from build123d import *
from build123d.topology import SkipClean

# Parameters (mm, degrees)
BOSS_EXTRUDE1_DEPTH = 5
SKETCH3_W           = 36.405926788
SKETCH3_H           = 27.783470444
CUT_EXTRUDE1_DEPTH  = 36
CUT_EXTRUDE2_REACH  = 86.1
SKETCH4_R           = 7.5
BOSS_EXTRUDE2_REACH = 86.1
SKETCH5_R           = 1
RIB2_REACH          = 70.337
SKETCH6_WALL_W      = 155.225095754
SKETCH6_WALL_H      = 3
RIB3_REACH          = 83.817
SKETCH7_WALL_W      = 192.357197592
SKETCH7_WALL_H      = 3
RIB4_REACH          = 83.817
SKETCH9_WALL_W      = 192.357197592
SKETCH9_WALL_H      = 3
SKETCH10_R          = 1.5
CUT_EXTRUDE3_DEPTH  = 5


with BuildPart() as part:
    # Sketch1 → Boss-Extrude1 (new body)
    with BuildSketch(Plane(origin=(0, 0, 0), x_dir=(1, 0, 0), z_dir=(0, 1, 0))):
        with BuildLine():
            Line((35, 20), (-35, 20))
            ThreePointArc((-35, 20), (-45.606601718, 15.606601718), (-50, 5))
            Line((-50, 5), (-50, -5))
            ThreePointArc((-50, -5), (-45.606601718, -15.606601718), (-35, -20))
            Line((-35, -20), (35, -20))
            ThreePointArc((35, -20), (45.606601718, -15.606601718), (50, -5))
            Line((50, -5), (50, 5))
            ThreePointArc((50, 5), (45.606601718, 15.606601718), (35, 20))
        make_face()
    extrude(amount=BOSS_EXTRUDE1_DEPTH)

    # Sketch2 → Revolve2 (revolve)
    with SkipClean():  # the faces are left unmerged after this step: merging them gives an invalid solid
        with BuildSketch(Plane.XY, mode=Mode.PRIVATE) as revolve2_sk:
            Polygon((-30, 0), (12.071067812, 42.071067812), (19.142135624, 35), (-15.857864376, 0), align=None)
        revolve(revolve2_sk.sketch.rotate(Axis((19.142135624, 35, 0), (-0.7071067811865515, -0.7071067811865436, 0)), 180), axis=Axis((19.142135624, 35, 0), (-0.7071067811865515, -0.7071067811865436, 0)))

    # Sketch3 → Cut-Extrude1 (cut)
    with BuildSketch(Plane.XZ):
        with Locations((-14.157860418, 0)):
            Rectangle(SKETCH3_W, SKETCH3_H)
    extrude(amount=CUT_EXTRUDE1_DEPTH, mode=Mode.SUBTRACT)

    # Cut-Extrude2: up to this plane
    cut_extrude2_end = Plane(origin=(-35, 5, -5), z_dir=(0, 1, 0))
    # Sketch4 → Cut-Extrude2 (cut, up to the surface)
    with BuildSketch(Plane(origin=(27.071067812, 27.071067812, 0), x_dir=(0, 0, -1), z_dir=(0.7071067811865513, 0.7071067811865438, 0)), mode=Mode.PRIVATE) as cut_extrude2_sk1:
        with Locations(Location((0, 11.213203436, 0), (0, 0, 90))):
            Circle(SKETCH4_R)
    cut_extrude2_tool1 = split(extrude(cut_extrude2_sk1.sketch, amount=-CUT_EXTRUDE2_REACH, mode=Mode.PRIVATE), bisect_by=cut_extrude2_end, keep=Keep.BOTH, mode=Mode.PRIVATE)
    add(cut_extrude2_tool1.solids().sort_by_distance((19.142136, 35, 0))[0], mode=Mode.SUBTRACT)

    # Boss-Extrude2: up to this plane
    boss_extrude2_end = Plane(origin=(-35, 5, -5), z_dir=(0, 1, 0))
    # Sketch5 → Boss-Extrude2 (add, up to the surface)
    with BuildSketch(Plane(origin=(27.071067812, 27.071067812, 0), x_dir=(0, 0, -1), z_dir=(0.7071067811865513, 0.7071067811865438, 0)), mode=Mode.PRIVATE) as boss_extrude2_sk1:
        with Locations((7.5, 11.213203436)):
            Circle(SKETCH5_R)
    boss_extrude2_tool1 = split(extrude(boss_extrude2_sk1.sketch, amount=-BOSS_EXTRUDE2_REACH, mode=Mode.PRIVATE), bisect_by=boss_extrude2_end, keep=Keep.BOTH, mode=Mode.PRIVATE)
    add(boss_extrude2_tool1.solids().sort_by_distance((19.142136, 35, -7.5))[0])
    # Sketch5 → Boss-Extrude2 (add, up to the surface)
    with BuildSketch(Plane(origin=(27.071067812, 27.071067812, 0), x_dir=(0, 0, -1), z_dir=(0.7071067811865513, 0.7071067811865438, 0)), mode=Mode.PRIVATE) as boss_extrude2_sk2:
        with Locations((5.303300859, 5.909902577)):
            Circle(SKETCH5_R)
    boss_extrude2_tool2 = split(extrude(boss_extrude2_sk2.sketch, amount=-BOSS_EXTRUDE2_REACH, mode=Mode.PRIVATE), bisect_by=boss_extrude2_end, keep=Keep.BOTH, mode=Mode.PRIVATE)
    add(boss_extrude2_tool2.solids().sort_by_distance((22.892136, 31.25, -5.303301))[0])
    # Sketch5 → Boss-Extrude2 (add, up to the surface)
    with BuildSketch(Plane(origin=(27.071067812, 27.071067812, 0), x_dir=(0, 0, -1), z_dir=(0.7071067811865513, 0.7071067811865438, 0)), mode=Mode.PRIVATE) as boss_extrude2_sk3:
        with Locations((0, 3.713203436)):
            Circle(SKETCH5_R)
    boss_extrude2_tool3 = split(extrude(boss_extrude2_sk3.sketch, amount=-BOSS_EXTRUDE2_REACH, mode=Mode.PRIVATE), bisect_by=boss_extrude2_end, keep=Keep.BOTH, mode=Mode.PRIVATE)
    add(boss_extrude2_tool3.solids().sort_by_distance((24.445436, 29.696699, 0))[0])
    # Sketch5 → Boss-Extrude2 (add, up to the surface)
    with BuildSketch(Plane(origin=(27.071067812, 27.071067812, 0), x_dir=(0, 0, -1), z_dir=(0.7071067811865513, 0.7071067811865438, 0)), mode=Mode.PRIVATE) as boss_extrude2_sk4:
        with Locations((-5.303300859, 5.909902577)):
            Circle(SKETCH5_R)
    boss_extrude2_tool4 = split(extrude(boss_extrude2_sk4.sketch, amount=-BOSS_EXTRUDE2_REACH, mode=Mode.PRIVATE), bisect_by=boss_extrude2_end, keep=Keep.BOTH, mode=Mode.PRIVATE)
    add(boss_extrude2_tool4.solids().sort_by_distance((22.892136, 31.25, 5.303301))[0])
    # Sketch5 → Boss-Extrude2 (add, up to the surface)
    with BuildSketch(Plane(origin=(27.071067812, 27.071067812, 0), x_dir=(0, 0, -1), z_dir=(0.7071067811865513, 0.7071067811865438, 0)), mode=Mode.PRIVATE) as boss_extrude2_sk5:
        with Locations((-7.5, 11.213203436)):
            Circle(SKETCH5_R)
    boss_extrude2_tool5 = split(extrude(boss_extrude2_sk5.sketch, amount=-BOSS_EXTRUDE2_REACH, mode=Mode.PRIVATE), bisect_by=boss_extrude2_end, keep=Keep.BOTH, mode=Mode.PRIVATE)
    add(boss_extrude2_tool5.solids().sort_by_distance((19.142136, 35, 7.5))[0])
    # Sketch5 → Boss-Extrude2 (add, up to the surface)
    with BuildSketch(Plane(origin=(27.071067812, 27.071067812, 0), x_dir=(0, 0, -1), z_dir=(0.7071067811865513, 0.7071067811865438, 0)), mode=Mode.PRIVATE) as boss_extrude2_sk6:
        with Locations((-5.303300859, 16.516504294)):
            Circle(SKETCH5_R)
    boss_extrude2_tool6 = split(extrude(boss_extrude2_sk6.sketch, amount=-BOSS_EXTRUDE2_REACH, mode=Mode.PRIVATE), bisect_by=boss_extrude2_end, keep=Keep.BOTH, mode=Mode.PRIVATE)
    add(boss_extrude2_tool6.solids().sort_by_distance((15.392136, 38.75, 5.303301))[0])
    # Sketch5 → Boss-Extrude2 (add, up to the surface)
    with BuildSketch(Plane(origin=(27.071067812, 27.071067812, 0), x_dir=(0, 0, -1), z_dir=(0.7071067811865513, 0.7071067811865438, 0)), mode=Mode.PRIVATE) as boss_extrude2_sk7:
        with Locations((0, 18.713203436)):
            Circle(SKETCH5_R)
    boss_extrude2_tool7 = split(extrude(boss_extrude2_sk7.sketch, amount=-BOSS_EXTRUDE2_REACH, mode=Mode.PRIVATE), bisect_by=boss_extrude2_end, keep=Keep.BOTH, mode=Mode.PRIVATE)
    add(boss_extrude2_tool7.solids().sort_by_distance((13.838835, 40.303301, 0))[0])
    # Sketch5 → Boss-Extrude2 (add, up to the surface)
    with BuildSketch(Plane(origin=(27.071067812, 27.071067812, 0), x_dir=(0, 0, -1), z_dir=(0.7071067811865513, 0.7071067811865438, 0)), mode=Mode.PRIVATE) as boss_extrude2_sk8:
        with Locations((5.303300859, 16.516504294)):
            Circle(SKETCH5_R)
    boss_extrude2_tool8 = split(extrude(boss_extrude2_sk8.sketch, amount=-BOSS_EXTRUDE2_REACH, mode=Mode.PRIVATE), bisect_by=boss_extrude2_end, keep=Keep.BOTH, mode=Mode.PRIVATE)
    add(boss_extrude2_tool8.solids().sort_by_distance((15.392136, 38.75, -5.303301))[0])

    # Sketch6 wall → Rib2 (add, up to next)
    with BuildSketch(Plane(origin=(26.502692564, 15.5, 0), x_dir=(0.422618261725, -0.906307787044, 0), z_dir=(0.906307787044, 0.422618261725, 0)), mode=Mode.PRIVATE) as rib2_sk1:
        Rectangle(SKETCH6_WALL_W, SKETCH6_WALL_H)
    rib2_tool1 = extrude(rib2_sk1.sketch, amount=-RIB2_REACH, mode=Mode.PRIVATE) - part.part
    add(rib2_tool1.solids().sort_by_distance((26.502692564, 15.5, 0))[0])

    # Sketch7 wall → Rib3 (add, up to next)
    with BuildSketch(Plane(origin=(17.261595026, 14.641447257, 10.75), x_dir=(0, -0.721603754863, 0.69230630574), z_dir=(0, -0.69230630574, -0.721603754863)), mode=Mode.PRIVATE) as rib3_sk1:
        Rectangle(SKETCH7_WALL_W, SKETCH7_WALL_H)
    rib3_tool1 = extrude(rib3_sk1.sketch, amount=RIB3_REACH, mode=Mode.PRIVATE) - part.part
    add(rib3_tool1.solids().sort_by_distance((17.261595026, 14.641447257, 10.75))[0])

    # Sketch9 wall → Rib4 (add, up to next)
    with BuildSketch(Plane(origin=(17.261595026, 14.641447257, -10.75), x_dir=(0, -0.721603754863, -0.69230630574), z_dir=(0, 0.69230630574, -0.721603754863)), mode=Mode.PRIVATE) as rib4_sk1:
        Rectangle(SKETCH9_WALL_W, SKETCH9_WALL_H)
    rib4_tool1 = extrude(rib4_sk1.sketch, amount=-RIB4_REACH, mode=Mode.PRIVATE) - part.part
    add(rib4_tool1.solids().sort_by_distance((17.261595026, 14.641447257, -10.75))[0])

    # Sketch10 → Cut-Extrude3 (cut)
    with BuildSketch(Plane.XZ):
        with Locations(Location((-40, 0, 0), (0, 0, 270))):
            Circle(SKETCH10_R)
        with Locations(Location((40, 15, 0), (0, 0, 270))):
            Circle(SKETCH10_R)
        with Locations(Location((40, -15, 0), (0, 0, 270))):
            Circle(SKETCH10_R)
    extrude(amount=-CUT_EXTRUDE3_DEPTH, mode=Mode.SUBTRACT)


solid = part.part
The listing builds one solid part. Answer for the finished solid, in the listing's coordinates (mm). A direction names the side the tool comes from. Give positions to 0.01 mm unless a question says otherwise; leave off trailing zeros. Order: outer loops, then holes, each group sorted by start corner. A loop starts at its lowest first (then second) coordinate and runs counter-clockwise, first axis right, second up. Notation, with made-up numbers: (-11, 52.25) - (33, 52.25) arc R20 cw to (33, 61.25) - close; hole circle Ø5 at (69, 4.25). An arc over 180 degrees is marked (long way). Use one line per item in the form item = value.
1) Find section D-D on z = 15. Determine the outline of the cut face in (x, y).
Verdict:
outline = (-46.18, 0) - (38.5, 0) - (38.5, 5) - (18.76, 5) - (18.76, 10.21) - (15.76, 10.21) - (15.76, 5) - (-46.18, 5) - close; (41.5, 0) - (46.18, 0) - (46.18, 5) - (41.5, 5) - close
2) Find section B-B on x = 40. Determine the outline of the cut face in (y, z), and give its area (3 significant figures).
Verdict:
outline = (0, -19.14) - (5, -19.14) - (5, -16.5) - (0, -16.5) - close; (0, -13.5) - (5, -13.5) - (5, 13.5) - (0, 13.5) - close; (0, 16.5) - (5, 16.5) - (5, 19.14) - (0, 19.14) - close
area = 161 mm^2
3) Consider probe 1 along X at (y, z) = (1.7, 0); probe 2 along Y at (x, z) = (14, 14); probe 3 along X at (y, z) = (2.35, 15). Determine where each line is inside the solid, lowest interval first. Write a range as [from, to].
Verdict:
probe_1 = [-50, -41.5], [-38.5, 50]
probe_2 = [0, 5]
probe_3 = [-46.18, 38.5], [41.5, 46.18]
4) The mould has two halves that part along X. Classify faces 1 (the cylindrical face through (11.323, 17.396, 2.895)), 2 (the flat face through (18.762, 10, -8)), 3 (the flat face through (-1, 0, 0)): released by +X, released by -X, zero draft, split by the parting line, or undercut.
Verdict:
face_1 = undercut
face_2 = released by +X
face_3 = zero draft
5) Find section A-A on z = 0. Determine the outline of the cut face in (x, y), and give its area (3 significant figures).
Verdict:
outline = (-50, 0) - (-41.5, 0) - (-41.5, 5) - (-50, 5) - close; (-38.5, 0) - (50, 0) - (50, 5) - (31.4, 5) - (22.46, 24.17) - (26.21, 27.93) - (23.74, 30.4) - (-1.67, 5) - (-20.05, 5) - (14.55, 39.6) - (12.07, 42.07) - (-25, 5) - (-38.5, 5) - close
area = 1,050 mm^2
6) For faces 4 (the flat face through (12, 10, 1.5)), 5 (the flat face through (-25, 5, -5)), 6 (the flat face through (12, 10, -1.5)), determine the directions among +Z, -Z, +X, -X, +Y, -Y from which every point of the face is accessible in a straight line to the end or side of a thin tool.
Verdict:
face_4 = +Z
face_5 = none
face_6 = -Z
7) Each of these flat-tipped pins is pushed along its axis until it touches: pin 1 (6 mm diameter, centred on y = 10, z = 7, fed in from +X); pin 2 (10 mm diameter, centred on x = -2, y = 26, fed in from -Z) (3 decimals); pin 3 (16.5 mm diameter, centred on x = -13, z = 0, fed in from +Y); pin 4 (2.5 mm diameter, centred on x = 40, z = -15, fed in from -Y). Where does it stop, or does it pass through?
Verdict:
pin_1 = 18.76
pin_2 = -9.335
pin_3 = 25.25
pin_4 = through
8) Find section C-C on x = -40. Determine the outline of the cut face in (y, z).
Verdict:
outline = (0, -19.14) - (5, -19.14) - (5, -1.5) - (0, -1.5) - close; (0, 1.5) - (5, 1.5) - (5, 19.14) - (0, 19.14) - close
